Geometry check sheet. Reference: the model listing, model coordinates, mm. Face numbers are marked on the shaded views. A direction names the side the tool comes from. Give positions to 0.01 mm unless a question says otherwise; leave off trailing zeros. Loops run counter-clockwise (first coordinate to the right, second up) from the corner with the lowest first, then second, coordinate; pieces in that order, holes last.
```python
from build123d import *
from build123d.topology import SkipClean

# Parameters (mm, degrees)
SKETCH1_R           = 11.984375
SKETCH1_R_2         = 1.984375
SKETCH1_R_3         = 0.75
BOSS_EXTRUDE1_DEPTH = 2
SKETCH6_W           = 23.96875
SKETCH6_H           = 8
CUT_EXTRUDE1_DEPTH  = 19.741677841
BOSS_EXTRUDE3_START = -2
SKETCH7_R           = 1.65
BOSS_EXTRUDE3_DEPTH = 2
SKETCH8_R           = 1.1
BOSS_EXTRUDE4_DEPTH = 1


with BuildPart() as part:
    # Sketch1 → Boss-Extrude1 (new body)
    with BuildSketch(Plane(origin=(0, 0, 0), x_dir=(1, 0, 0), z_dir=(0, 1, 0))):
        with Locations(Location((0, 0, 0), (0, 0, 270))):
            Circle(SKETCH1_R)
        with Locations(Location((0, 0, 0), (0, 0, 270))):
            Circle(SKETCH1_R_2, mode=Mode.SUBTRACT)
        with Locations(Location((0, 10, 0), (0, 0, 270))):
            Circle(SKETCH1_R_3, mode=Mode.SUBTRACT)
        with Locations(Location((5.877852523, 8.090169944, 0), (0, 0, 270))):
            Circle(SKETCH1_R_3, mode=Mode.SUBTRACT)
        with Locations(Location((9.510565163, 3.090169944, 0), (0, 0, 270))):
            Circle(SKETCH1_R_3, mode=Mode.SUBTRACT)
        with Locations(Location((9.510565163, -3.090169944, 0), (0, 0, 270))):
            Circle(SKETCH1_R_3, mode=Mode.SUBTRACT)
        with Locations(Location((5.877852523, -8.090169944, 0), (0, 0, 270))):
            Circle(SKETCH1_R_3, mode=Mode.SUBTRACT)
        with Locations(Location((0, -10, 0), (0, 0, 270))):
            Circle(SKETCH1_R_3, mode=Mode.SUBTRACT)
        with Locations(Location((-5.877852523, -8.090169944, 0), (0, 0, 270))):
            Circle(SKETCH1_R_3, mode=Mode.SUBTRACT)
        with Locations(Location((-9.510565163, -3.090169944, 0), (0, 0, 270))):
            Circle(SKETCH1_R_3, mode=Mode.SUBTRACT)
        with Locations(Location((-9.510565163, 3.090169944, 0), (0, 0, 270))):
            Circle(SKETCH1_R_3, mode=Mode.SUBTRACT)
        with Locations(Location((-5.877852523, 8.090169944, 0), (0, 0, 270))):
            Circle(SKETCH1_R_3, mode=Mode.SUBTRACT)
    extrude(amount=BOSS_EXTRUDE1_DEPTH)

    # Sweep1: sweep along a path in Sketch3
    with SkipClean():  # the faces are left unmerged after this step: merging them gives an invalid solid
        with BuildLine(Plane(origin=(0, 0, 0), x_dir=(0, 0, -1), z_dir=(1, 0, 0))) as sweep1_path:
            Line((0, 2), (0, 8))
        # Sketch2 → Sweep1 (sweep)
        with BuildSketch(Plane(origin=(0, 2, 0), x_dir=(1, 0, 0), z_dir=(0, 1, 0))):
            with BuildLine():
                Line((-0.5, 9.236476601), (-0.5, 1.920350005))
                ThreePointArc((-0.5, 1.920350005), (-0.613205598, 1.887252775), (-0.724244915, 1.847488415))
                Line((-0.724244915, 1.847488415), (-5.024556232, 7.766359164))
                ThreePointArc((-5.024556232, 7.766359164), (-2.858407198, 8.797272776), (-0.5, 9.236476601))
            make_face()
            with BuildLine():
                Line((0.5, 9.236476601), (0.5, 1.920350005))
                ThreePointArc((0.5, 1.920350005), (0.613205598, 1.887252775), (0.724244915, 1.847488415))
                Line((0.724244915, 1.847488415), (5.024556232, 7.766359164))
                ThreePointArc((5.024556232, 7.766359164), (2.858407198, 8.797272776), (0.5, 9.236476601))
            make_face()
            with BuildLine():
                Line((5.833573226, 7.178573912), (1.533261909, 1.259703163))
                ThreePointArc((1.533261909, 1.259703163), (1.605393098, 1.16638636), (1.671852888, 1.068949045))
                Line((1.671852888, 1.068949045), (8.629902762, 3.329756496))
                ThreePointArc((8.629902762, 3.329756496), (7.483407198, 5.437013584), (5.833573226, 7.178573912))
            make_face()
            with BuildLine():
                Line((8.938919756, 2.37869998), (1.980869883, 0.117892528))
                ThreePointArc((1.980869883, 0.117892528), (1.984375, 0), (1.980869883, -0.117892528))
                Line((1.980869883, -0.117892528), (8.938919756, -2.37869998))
                ThreePointArc((8.938919756, -2.37869998), (9.25, 0), (8.938919756, 2.37869998))
            make_face()
            with BuildLine():
                Line((8.629902762, -3.329756496), (1.671852888, -1.068949045))
                ThreePointArc((1.671852888, -1.068949045), (1.605393098, -1.16638636), (1.533261909, -1.259703163))
                Line((1.533261909, -1.259703163), (5.833573226, -7.178573912))
                ThreePointArc((5.833573226, -7.178573912), (7.483407198, -5.437013584), (8.629902762, -3.329756496))
            make_face()
            with BuildLine():
                Line((5.024556232, -7.766359164), (0.724244915, -1.847488415))
                ThreePointArc((0.724244915, -1.847488415), (0.613205598, -1.887252775), (0.5, -1.920350005))
                Line((0.5, -1.920350005), (0.5, -9.236476601))
                ThreePointArc((0.5, -9.236476601), (2.858407198, -8.797272776), (5.024556232, -7.766359164))
            make_face()
            with BuildLine():
                Line((-0.5, -9.236476601), (-0.5, -1.920350005))
                ThreePointArc((-0.5, -1.920350005), (-0.613205598, -1.887252775), (-0.724244915, -1.847488415))
                Line((-0.724244915, -1.847488415), (-5.024556232, -7.766359164))
                ThreePointArc((-5.024556232, -7.766359164), (-2.858407198, -8.797272776), (-0.5, -9.236476601))
            make_face()
            with BuildLine():
                Line((-5.833573226, -7.178573912), (-1.533261909, -1.259703163))
                ThreePointArc((-1.533261909, -1.259703163), (-1.605393098, -1.16638636), (-1.671852888, -1.068949045))
                Line((-1.671852888, -1.068949045), (-8.629902762, -3.329756496))
                ThreePointArc((-8.629902762, -3.329756496), (-7.483407198, -5.437013584), (-5.833573226, -7.178573912))
            make_face()
            with BuildLine():
                Line((-8.938919756, -2.37869998), (-1.980869883, -0.117892528))
                ThreePointArc((-1.980869883, -0.117892528), (-1.984375, 0), (-1.980869883, 0.117892528))
                Line((-1.980869883, 0.117892528), (-8.938919756, 2.37869998))
                ThreePointArc((-8.938919756, 2.37869998), (-9.25, 0), (-8.938919756, -2.37869998))
            make_face()
            with BuildLine():
                Line((-8.629902762, 3.329756496), (-1.671852888, 1.068949045))
                ThreePointArc((-1.671852888, 1.068949045), (-1.605393098, 1.16638636), (-1.533261909, 1.259703163))
                Line((-1.533261909, 1.259703163), (-5.833573226, 7.178573912))
                ThreePointArc((-5.833573226, 7.178573912), (-7.483407198, 5.437013584), (-8.629902762, 3.329756496))
            make_face()
        sweep(path=sweep1_path.line)

    # Sketch4 → Revolve1 (revolve)
    with SkipClean():  # the faces are left unmerged after this step: merging them gives an invalid solid
        with BuildSketch(Plane(origin=(0, 0, 0), x_dir=(0, 0, -1), z_dir=(1, 0, 0)), mode=Mode.PRIVATE) as revolve1_sk:
            Polygon((-2.37869998, 2), (-1.984375, 2), (-1.984375, 8), align=None)
        revolve(revolve1_sk.sketch.rotate(Axis((0, 0, 0), (0, 1, 0)), 165.405971265), axis=Axis((0, 0, 0), (0, 1, 0)))

    # Sketch6 → Cut-Extrude1 (cut, through all)
    with SkipClean():  # the faces are left unmerged after this step: merging them gives an invalid solid
        with BuildSketch(Plane(origin=(0, 0, 0), x_dir=(-0.3193728209047868, 0, -0.9476291475399641), z_dir=(-0.9476291475399641, 0, 0.3193728209047868))):
            with Locations((0, -4)):
                Rectangle(SKETCH6_W, SKETCH6_H)
        extrude(amount=-CUT_EXTRUDE1_DEPTH, mode=Mode.SUBTRACT)

    # Sketch7 → Boss-Extrude3 (add)
    with SkipClean():  # the faces are left unmerged after this step: merging them gives an invalid solid
        with BuildSketch(Plane(origin=(0, 2, 0), x_dir=(1, 0, 0), z_dir=(0, 1, 0)).offset(BOSS_EXTRUDE3_START)):
            with BuildLine():
                Line((-9.021857716, -7.888683508), (-1.576209535, -16.403865848))
                ThreePointArc((-1.576209535, -16.403865848), (2.803074288, -17.134270389), (4.375298385, -12.982195127))
                Line((4.375298385, -12.982195127), (3.827483651, -11.356743065))
                ThreePointArc((3.827483651, -11.356743065), (-3.122857627, -11.570350227), (-9.021857716, -7.888683508))
            make_face()
            with Locations(Location((1.058596369, -14.1, 0), (0, 0, 270))):
                Circle(SKETCH7_R, mode=Mode.SUBTRACT)
        extrude(amount=BOSS_EXTRUDE3_DEPTH)

    # Sketch8 → Boss-Extrude4 (add)
    # profile 1 of 2: a face of its own
    with SkipClean():  # the faces are left unmerged after this step: merging them gives an invalid solid
        with BuildSketch(Plane(origin=(0, 0, 0), x_dir=(-0.31937282090478675, 0, -0.9476291475399641), z_dir=(0.9476291475399641, 0, -0.31937282090478675))):
            with BuildLine():
                Line((-13.25, 4), (-13.25, 2))
                Line((-13.25, 2), (-8.75, 2))
                Line((-8.75, 2), (-8.75, 6.5))
                Line((-8.75, 6.5), (-9.25, 6.5))
                Line((-9.25, 6.5), (-10.75, 6.5))
                ThreePointArc((-10.75, 6.5), (-12.517766953, 5.767766953), (-13.25, 4))
            make_face()
            with Locations((-10.75, 4)):
                Circle(SKETCH8_R, mode=Mode.SUBTRACT)
        # profile 2 of 2: a face of its own
        with BuildSketch(Plane(origin=(0, 0, 0), x_dir=(-0.31937282090478675, 0, -0.9476291475399641), z_dir=(0.9476291475399641, 0, -0.31937282090478675))):
            with BuildLine():
                Line((11.484375, 2), (8.75, 2))
                Line((8.75, 2), (8.75, 6.5))
                Line((8.75, 6.5), (9.25, 6.5))
                Line((9.25, 6.5), (10.75, 6.5))
                ThreePointArc((10.75, 6.5), (12.517766953, 5.767766953), (13.25, 4))
                Line((13.25, 4), (13.25, 2))
                Line((13.25, 2), (13.25, 0))
                Line((13.25, 0), (11.984375, 0))
                Line((11.984375, 0), (11.484375, 0))
                Line((11.484375, 0), (11.484375, 2))
            make_face()
            with Locations((10.75, 4)):
                Circle(SKETCH8_R, mode=Mode.SUBTRACT)
        extrude(amount=-BOSS_EXTRUDE4_DEPTH)


solid = part.part
```
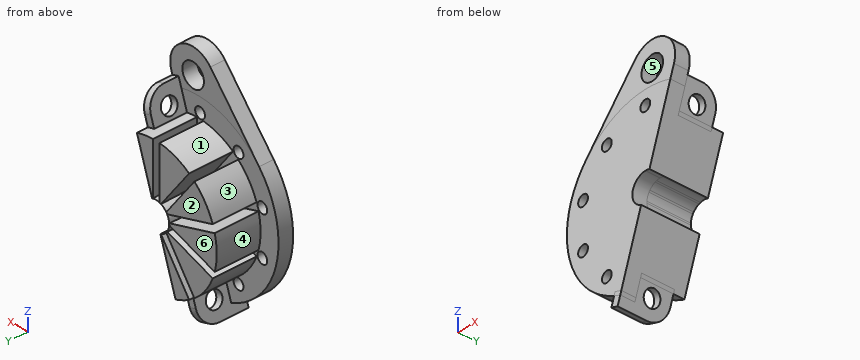
1) Sectioned sample at B-B on y = 7. Enter the section's corners in (x, z), plus the area to 3 significant figures.
2) Scan lines: line 1 along Z through (x, y) = (-7, 6.25); line 2 along Z through (x, y) = (-6.25, 2.25); line 3 along Z through (x, y) = (-3.75, 7.5). Record each from-to range of solid material in increasing order.
3) Mould release check, pull along Z, two halves, no side actions. Record for the marked faces 3, 4, 5 and 6: +Z half, -Z half, draft (parallel to the pull), parting line (faces both ways), or undercut.
4) Depth check by flat-ended pin: P1, Ø3, axis at x = -5, y = 5.5, coming from the -Z side; P2, Ø4, axis at y = 3, z = 4.5, coming from the -X side; P3, Ø1.5, axis at y = 4.5, z = -4.5, coming from the +X side. Enter the tip coordinate at first touch or a pass-through.
5) Sectioned sample at A-A on z = 14.1. Enter the section's corners in (x, y).
6) Sectioned sample at C-C on x = -11. Enter the section's corners in (y, z).
7) Tool access check on the marked faces 1 and 2. Record the directions out of +Z, -Z, +X, -X, +Y, -Y that give a thin tool (end or side, any length) a straight path to the whole face; none if there is none.
Determined:
1. outline: (-8.94, -2.38) - (-2.05, -0.14) arc R2.05 ccw to (-1.74, -1.09) - (-8.63, -3.33) arc R9.25 ccw to (-5.83, -7.18) - (-1.57, -1.31) arc R2.05 ccw to (-0.76, -1.9) - (-5.02, -7.77) arc R9.25 ccw to (-2.95, -8.77) - (-0.63, -1.88) arc R1.98 cw to (0.63, 1.88) - (2.95, 8.77) arc R9.25 ccw to (0.5, 9.24) - (0.5, 1.99) arc R2.05 ccw to (-0.5, 1.99) - (-0.5, 9.24) arc R9.25 ccw to (-5.02, 7.77) - (-0.76, 1.9) arc R2.05 ccw to (-1.57, 1.31) - (-5.83, 7.18) arc R9.25 ccw to (-8.63, 3.33) - (-1.74, 1.09) arc R2.05 ccw to (-2.05, 0.14) - (-8.94, 2.38) arc R9.25 ccw to start
1. area: 92.1 mm2
2. line 1: z = -6.05 to -2.8, -1.75 to 1.75, 2.8 to 6.05
2. line 2: z = -6.82 to -2.56, -1.51 to 1.51, 2.56 to 6.82
2. line 3: z = -8.46 to -6.01, -4.31 to -1.74, -0.69 to 0.69, 1.74 to 4.31, 6.01 to 8.46
3. face 3: +Z half
3. face 4: parting line
3. face 5: undercut
3. face 6: draft
4. P1: stops at z = -12.55
4. P2: stops at x = -11.66
4. P3: stops at x = -1.26
5. outline: (-3.59, 0) - (-0.59, 0) - (-0.59, 2) - (-3.59, 2) - close; (2.71, 0) - (4.56, 0) - (4.56, 2) - (2.71, 2) - close
6. outline: (0, -4.76) - (2, -4.76) - (2, 4.76) - (0, 4.76) - close
7. face 1: +Z, -X, +Y
7. face 2: +Z, -Z, +X, -X, +Y
